```python
from build123d import *

# Parameters (mm, degrees)
F0_R     = 9.525
F1_DEPTH = 25.4
F3_DEPTH = 25.4
F5_DEPTH = 25.401
F6_DEPTH = 9.525
F8_DEPTH = 12.7


with BuildPart() as f1:
    # F0 (on Front) → F1 (new body)
    with BuildSketch(Plane.XZ):
        Circle(F0_R)
    extrude(amount=F1_DEPTH)

    # F2 (on Front) → F3 (join)
    with BuildSketch(Plane.XZ):
        with BuildLine():
            Line((0, -4.7625), (4.7625, -4.7625))
            Line((4.7625, -4.7625), (4.7625, 0))
            ThreePointArc((4.7625, 0), (3.367596, -3.367596), (0, -4.7625))
        make_face()
        with BuildLine():
            Line((-4.7625, -4.7625), (0, -4.7625))
            ThreePointArc((0, -4.7625), (-3.367596, -3.367596), (-4.7625, 0))
            Line((-4.7625, 0), (-4.7625, -4.7625))
        make_face()
        with BuildLine():
            ThreePointArc((0, 4.7625), (3.367596, 3.367596), (4.7625, 0))
            Line((4.7625, 0), (4.7625, 4.7625))
            Line((4.7625, 4.7625), (0, 4.7625))
        make_face()
        with BuildLine():
            Line((-4.7625, 4.7625), (-4.7625, 0))
            ThreePointArc((-4.7625, 0), (-3.367596, 3.367596), (0, 4.7625))
            Line((0, 4.7625), (-4.7625, 4.7625))
        make_face()
    extrude(amount=F3_DEPTH)

    # F4 (on Front) → F5 (cut, through all)
    with BuildSketch(Plane.XZ):
        with BuildLine():
            ThreePointArc((-4.7625, 0), (-3.367596, -3.367596), (0, -4.7625))
            ThreePointArc((0, -4.7625), (3.367596, -3.367596), (4.7625, 0))
            ThreePointArc((4.7625, 0), (3.367596, 3.367596), (0, 4.7625))
            ThreePointArc((0, 4.7625), (-3.367596, 3.367596), (-4.7625, 0))
        make_face()
    extrude(amount=F5_DEPTH, mode=Mode.SUBTRACT)

    # F4 (on Front) → F6 (cut)
    with BuildSketch(Plane.XZ):
        with BuildLine():
            Line((0, -4.7625), (4.7625, -4.7625))
            Line((4.7625, -4.7625), (4.7625, 0))
            ThreePointArc((4.7625, 0), (3.367596, -3.367596), (0, -4.7625))
        make_face()
        with BuildLine():
            Line((-4.7625, -4.7625), (0, -4.7625))
            ThreePointArc((0, -4.7625), (-3.367596, -3.367596), (-4.7625, 0))
            Line((-4.7625, 0), (-4.7625, -4.7625))
        make_face()
        with BuildLine():
            ThreePointArc((0, 4.7625), (3.367596, 3.367596), (4.7625, 0))
            Line((4.7625, 0), (4.7625, 4.7625))
            Line((4.7625, 4.7625), (0, 4.7625))
        make_face()
        with BuildLine():
            Line((-4.7625, 4.7625), (-4.7625, 0))
            ThreePointArc((-4.7625, 0), (-3.367596, 3.367596), (0, 4.7625))
            Line((0, 4.7625), (-4.7625, 4.7625))
        make_face()
    extrude(amount=F6_DEPTH, mode=Mode.SUBTRACT)

    # F7 (on face) → F8 (cut)
    with BuildSketch(Plane(origin=(0, 0, 0), x_dir=(-1, 0, 0), z_dir=(0, 1, 0))):
        Polygon((7.14904, -4.1275), (7.14904, 4.1275), (0, 8.255), (-7.14904, 4.1275), (-7.14904, -4.1275), (0, -8.255), align=None)
    extrude(amount=-F8_DEPTH, mode=Mode.SUBTRACT)


solid = f1.part
```
Source: CAD feature listing. Evaluate the final solid. Frame: model axes, mm. A direction names the side the tool comes from. Give positions to 0.01 mm unless a question says otherwise; leave off trailing zeros. Write each loop counter-clockwise with the first axis right and the second up, starting at its lowest first coordinate (ties: lowest second). Pieces come first, ordered by that corner, then holes.
1. Section query A-A (z = -3.75). Return the cut outline in (x, y).
2. Access query for faces 5 (the face through (-3.625, -6.261, 6.162)), 6 (the face through (-4.4, -25.4, 2.3)). Directions: +Z, -Z, +X, -X, +Y, -Y. A direction counts if a zero-diameter tool reaches every point of the face in a straight line with its end or side. Return the directions, or none.
3. Pull-direction query (X, two-part tool) for faces 1 (the face through (3.524, -6.261, 6.22)), 2 (the face through (-3.6, 0, 6.4)), 3 (the face through (-3.524, -6.261, -6.22)), 4 (the face through (-7.559, -12.522, -5.796)); classes: +X half, -X half, draft (parallel to the pull), parting line (faces both ways), or undercut.
4. First-contact query: pin 1 (3 mm diameter, centred on x = -2, y = -21, fed in from -Z); pin 2 (6 mm diameter, centred on x = -5, y = -12, fed in from -Z); pin 3 (4 mm diameter, centred on x = 6, y = -15.5, fed in from -Z); pin 4 (5 mm diameter, centred on y = -19, z = 0.5, fed in from -X) (3 decimals). Flat tips, straight axial feed; report the tip coordinate or a pass-through.
5. Section query B-B (x = 2.25). Return the cut outline in (y, z), then the cut area to 3 significant figures.
6. Material intervals for line 1 along Y through (x, z) = (2, 7); line 2 along Z through (x, y) = (-1, -23.25); line 3 along X through (y, z) = (-9, -2.5), sorted ascending.
Output values:
1. outline: (-8.76, -25.4) - (-2.94, -25.4) - (-2.94, -12.7) - (-7.15, -12.7) - (-7.15, 0) - (-8.76, 0) - close; (2.94, -25.4) - (8.76, -25.4) - (8.76, 0) - (7.15, 0) - (7.15, -12.7) - (2.94, -12.7) - close
2. face 5: +Y
2. face 6: +Z, -Z, +X, -X, -Y
3. face 1: undercut
3. face 2: draft
3. face 3: undercut
3. face 4: parting line
4. pin 1: stops at z = -9.51
4. pin 2: stops at z = -9.31
4. pin 3: stops at z = -8.64
4. pin 4: stops at x = -9.525
5. outline: (-25.4, -9.26) - (0, -9.26) - (0, -6.96) - (-12.7, -6.96) - (-12.7, -4.2) - (-25.4, -4.2) - close; (-25.4, 4.2) - (-12.7, 4.2) - (-12.7, 6.96) - (0, 6.96) - (0, 9.26) - (-25.4, 9.26) - close
5. area: 187 mm2
6. line 1: y = -25.4 to -12.7
6. line 2: z = -9.47 to -4.66, 4.66 to 9.47
6. line 3: x = -9.19 to -7.15, 7.15 to 9.19
